Design review of the part built by this model. Coordinates are the model's own, in mm. A direction names the side the tool comes from. Coordinates: 2 decimals unless noted, no trailing zeros. Write each loop counter-clockwise with the first axis right and the second up, starting at its lowest first coordinate (ties: lowest second). Pieces come first, ordered by that corner, then holes.
```python
from build123d import *

# Parameters (mm, degrees)
SKETCH2_R          = 12.7
CUT_EXTRUDE1_DEPTH = 10


with BuildPart() as part:
    # Sketch1 → Revolve1 (revolve)
    with BuildSketch(Plane.XY, mode=Mode.PRIVATE) as revolve1_sk:
        Polygon((12.7, -4), (100, -4), (100, 1), (125, 1), (125, -19), (100, -19), (100, -14), (12.7, -14), align=None)
    revolve(revolve1_sk.sketch.rotate(Axis((0, 113.049804917, 0), (0, -1, 0)), 90), axis=Axis((0, 113.049804917, 0), (0, -1, 0)))

    # Sketch2 → Cut-Extrude1 (cut)
    with BuildSketch(Plane(origin=(0, -4, 0), x_dir=(1, 0, 0), z_dir=(0, 1, 0))):
        with Locations(Location((0, 61.801458798, 0), (0, 0, 270))):
            Circle(SKETCH2_R)
        with Locations(Location((53.52163331, 30.900729399, 0), (0, 0, 270))):
            Circle(SKETCH2_R)
        with Locations(Location((53.52163331, -30.900729399, 0), (0, 0, 270))):
            Circle(SKETCH2_R)
        with Locations(Location((0, -61.801458798, 0), (0, 0, 270))):
            Circle(SKETCH2_R)
        with Locations(Location((-53.52163331, -30.900729399, 0), (0, 0, 270))):
            Circle(SKETCH2_R)
        with Locations(Location((-53.52163331, 30.900729399, 0), (0, 0, 270))):
            Circle(SKETCH2_R)
    extrude(amount=-CUT_EXTRUDE1_DEPTH, mode=Mode.SUBTRACT)


solid = part.part
```
(1) Consider section B-B (z = 0). Give the boundary of the cut face in (x, y), plus the area to 3 significant figures.
(2) Mouldability with a two-part tool opening along Z and no side actions: class faces 4 (the cylindrical face through (-44.94, -8.93, -40.26)), 5 (the flat face through (-84, 1, 56)), 6 (the cylindrical face through (-5.5, -9.14, -124.88)) as +Z half, -Z half, draft (parallel to the pull), parting line (faces both ways), or undercut.
(3) Consider section C-C (z = -34). Give the boundary of the cut face in (x, y), plus the area to 3 significant figures.
(4) Insertion check: pin 1 Ø23 at (x, z) = (0, 0) entering from -Y; pin 2 Ø6 at (y, z) = (-11, 37) entering from -X; pin 3 Ø2 at (y, z) = (-9, 31) entering from -X; pin 4 Ø4 at (x, y) = (-30.5, -8.5) entering from +Z. Each pin has a flat end and moves straight along its axis. Give the tip position at first contact, or say it passes through.
(5) For faces 1 (the cylindrical face through (-40.93, -8.93, 29.25)), 2 (the flat face through (21, -4, 1)), 3 (the flat face through (21, -14, -1)), list the 3-axis set-ups (+Z, -Z, +X, -X, +Y, -Y) from which the entire face can be reached by the end or side of a thin tool; tool diameter is ignored.
(6) Consider section D-D (y = -9.5). Give the boundary of the cut face in (x, z), plus the area to 3 significant figures.
(7) Consider section A-A (x = 0). Give the boundary of the cut face in (y, z).
(8) Wall thickness on line 1 (X direction, y = -10.5, z = 0); line 2 (X direction, y = -7, z = 41.5); line 3 (X direction, y = -2.2, z = 0): over which ranges is each line inside the solid? List them lowest first.
Results:
1. outline: (-125, -19) - (-100, -19) - (-100, -14) - (-12.7, -14) - (-12.7, -4) - (-100, -4) - (-100, 1) - (-125, 1) - close; (12.7, -14) - (100, -14) - (100, -19) - (125, -19) - (125, 1) - (100, 1) - (100, -4) - (12.7, -4) - close
1. area: 2,750 mm2
2. face 4: undercut
2. face 5: draft
2. face 6: parting line
3. outline: (-120.29, -19) - (-94.04, -19) - (-94.04, -14) - (-65.84, -14) - (-65.84, -4) - (-94.04, -4) - (-94.04, 1) - (-120.29, 1) - close; (-41.21, -14) - (41.21, -14) - (41.21, -4) - (-41.21, -4) - close; (65.84, -14) - (94.04, -14) - (94.04, -19) - (120.29, -19) - (120.29, 1) - (94.04, 1) - (94.04, -4) - (65.84, -4) - close
3. area: 2,440 mm2
4. pin 1: passes through
4. pin 2: stops at x = -120.29
4. pin 3: stops at x = -121.35
4. pin 4: stops at z = 121.71
5. face 1: +Y, -Y
5. face 2: +Y
5. face 3: -Y
6. outline: circle Ø250 at (0, 0); hole circle Ø25.4 at (-53.52, -30.9); hole circle Ø25.4 at (-53.52, 30.9); hole circle Ø25.4 at (0, -61.8); hole circle Ø25.4 at (0, 0); hole circle Ø25.4 at (0, 61.8); hole circle Ø25.4 at (53.52, -30.9); hole circle Ø25.4 at (53.52, 30.9)
6. area: 45,500 mm2
7. outline: (-19, -125) - (1, -125) - (1, -100) - (-4, -100) - (-4, -74.5) - (-14, -74.5) - (-14, -100) - (-19, -100) - close; (-19, 100) - (-14, 100) - (-14, 74.5) - (-4, 74.5) - (-4, 100) - (1, 100) - (1, 125) - (-19, 125) - close; (-14, -49.1) - (-4, -49.1) - (-4, -12.7) - (-14, -12.7) - close; (-14, 12.7) - (-4, 12.7) - (-4, 49.1) - (-14, 49.1) - close
8. line 1: x = -125 to -12.7, 12.7 to 125
8. line 2: x = -117.91 to -60.52, -46.53 to 46.53, 60.52 to 117.91
8. line 3: x = -125 to -100, 100 to 125
